Build history of the part. All positions in model axes, mm. Face numbers are marked on the shaded views. A direction names the side the tool comes from. Coordinates: 2 decimals unless noted, no trailing zeros. Write each loop counter-clockwise with the first axis right and the second up, starting at its lowest first coordinate (ties: lowest second). Pieces come first, ordered by that corner, then holes.
```python
from build123d import *

# Parameters (mm, degrees)
SKETCH1_W           = 25
SKETCH1_H           = 52
BOSS_EXTRUDE1_DEPTH = 2
SKETCH2_W           = 25
SKETCH2_H           = 42.5
BOSS_EXTRUDE2_DEPTH = 2
SKETCH3_W           = 25
SKETCH3_H           = 42.5
BOSS_EXTRUDE3_DEPTH = 2
SKETCH4_R           = 2.5
CUT_EXTRUDE1_DEPTH  = 70
SKETCH5_R           = 4
CUT_EXTRUDE2_DEPTH  = 21
SKETCH6_R           = 1.5
CUT_EXTRUDE3_DEPTH  = 21


with BuildPart() as part:
    # Sketch1 → Boss-Extrude1 (new body)
    with BuildSketch(Plane.XY):
        with Locations((-0.174770451, 4.502942624)):
            Rectangle(SKETCH1_W, SKETCH1_H)
    extrude(amount=BOSS_EXTRUDE1_DEPTH)

    # Sketch2 → Boss-Extrude2 (add)
    with BuildSketch(Plane(origin=(0, 30.502942624, 0), x_dir=(1, 0, 0), z_dir=(0, 1, 0))):
        with Locations((-0.174770451, -21.25)):
            Rectangle(SKETCH2_W, SKETCH2_H)
    extrude(amount=BOSS_EXTRUDE2_DEPTH)

    # Sketch3 → Boss-Extrude3 (add)
    with BuildSketch(Plane(origin=(0, -21.497057376, 0), x_dir=(-1, 0, 0), z_dir=(0, -1, 0))):
        with Locations((0.174770451, -21.25)):
            Rectangle(SKETCH3_W, SKETCH3_H)
    extrude(amount=BOSS_EXTRUDE3_DEPTH)

    # Sketch4 → Cut-Extrude1 (cut)
    with BuildSketch(Plane(origin=(0, 32.502942624, 0), x_dir=(1, 0, 0), z_dir=(0, 1, 0))):
        with Locations(Location((-0.174770451, -32, 0), (0, 0, 90))):
            Circle(SKETCH4_R)
    extrude(amount=-CUT_EXTRUDE1_DEPTH, mode=Mode.SUBTRACT)

    # Sketch5 → Cut-Extrude2 (cut)
    with BuildSketch(Plane(origin=(0, 0, 0), x_dir=(-1, 0, 0), z_dir=(0, 0, -1))):
        with Locations((0.174770451, 4.502942624)):
            Circle(SKETCH5_R)
    extrude(amount=-CUT_EXTRUDE2_DEPTH, mode=Mode.SUBTRACT)

    # Sketch6 → Cut-Extrude3 (cut)
    with BuildSketch(Plane(origin=(0, 0, 0), x_dir=(-1, 0, 0), z_dir=(0, 0, -1))):
        with Locations((7.174770451, 4.502942624)):
            Circle(SKETCH6_R)
        with Locations((0.174770451, -2.497057376)):
            Circle(SKETCH6_R)
        with Locations((-6.825229549, 4.502942624)):
            Circle(SKETCH6_R)
        with Locations((0.174770451, 11.502942624)):
            Circle(SKETCH6_R)
    extrude(amount=-CUT_EXTRUDE3_DEPTH, mode=Mode.SUBTRACT)


solid = part.part
```
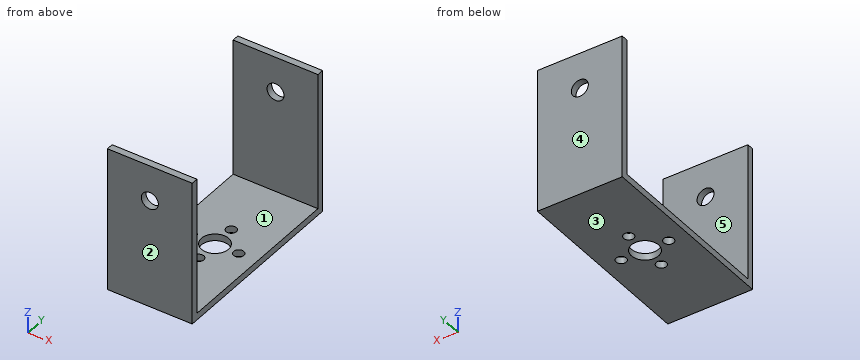
1. 3-axis set-ups, long thin cutter, end or side, ignore diameter. For the marked faces 4 and 5: which of +Z, -Z, +X, -X, +Y, -Y reach the whole face in a straight line?
Computed values:
face 4: +Z, -Z, +X, -X, +Y
face 5: +Z, +X, -X
2. Saw through at B-B on z = 22.5. List the corners of the cut face in (x, y), plus the area to 3 significant figures.
Computed values:
outline: (-12.67, -23.5) - (12.33, -23.5) - (12.33, -21.5) - (-12.67, -21.5) - close; (-12.67, 30.5) - (12.33, 30.5) - (12.33, 32.5) - (-12.67, 32.5) - close
area: 100 mm2
3. Mould opens along Y. For the marked faces 1, 2 and 3 say: +Y half, -Y half, draft (parallel to the pull), parting line (faces both ways), or undercut.
Computed values:
face 1: undercut
face 2: -Y half
face 3: draft
4. Saw through at C-C on x = 10. List the corners of the cut face in (y, z).
Computed values:
outline: (-23.5, 0) - (32.5, 0) - (32.5, 42.5) - (30.5, 42.5) - (30.5, 2) - (-21.5, 2) - (-21.5, 42.5) - (-23.5, 42.5) - close
5. Probe line 1 along Y through (x, z) = (9, 8.5); line 2 along X through (y, z) = (32, 32); line 3 along Z through (x, y) = (-10.25, 29.5). List the from-to ranges inside material, lowest first.
Computed values:
line 1: y = -23.5 to -21.5, 30.5 to 32.5
line 2: x = -12.67 to -2.67, 2.33 to 12.33
line 3: z = 0 to 2
6. Flat gauge pins, fed straight in: pin 1 (5 mm diameter, centred on x = -7.17, y = 4.5, fed in from +Z); pin 2 (2.5 mm diameter, centred on x = 6.83, y = 4.5, fed in from -Z). Where does each tip first touch, or does it go through?
Computed values:
pin 1: stops at z = 2
pin 2: passes through
7. Saw through at A-A on z = 32. List the corners of the cut face in (x, y), plus the area to 3 significant figures.
Computed values:
outline: (-12.67, -23.5) - (-2.67, -23.5) - (-2.67, -21.5) - (-12.67, -21.5) - close; (-12.67, 30.5) - (-2.67, 30.5) - (-2.67, 32.5) - (-12.67, 32.5) - close; (2.33, -23.5) - (12.33, -23.5) - (12.33, -21.5) - (2.33, -21.5) - close; (2.33, 30.5) - (12.33, 30.5) - (12.33, 32.5) - (2.33, 32.5) - close
area: 80.0 mm2
8. Saw through at D-D on x = 6.75. List the corners of the cut face in (y, z), plus the area to 3 significant figures.
Computed values:
outline: (-23.5, 0) - (3, 0) - (3, 2) - (-21.5, 2) - (-21.5, 42.5) - (-23.5, 42.5) - close; (6, 0) - (32.5, 0) - (32.5, 42.5) - (30.5, 42.5) - (30.5, 2) - (6, 2) - close
area: 268 mm2
